Check sheet for the modelled part. Datum: model origin and axes. Units: mm. A direction names the side the tool comes from. Give positions to 0.01 mm unless a question says otherwise; leave off trailing zeros. Loops run counter-clockwise (first coordinate to the right, second up) from the corner with the lowest first, then second, coordinate; pieces in that order, holes last.
```python
from build123d import *

# Parameters (mm, degrees)
SKETCH2_R           = 10
BOSS_EXTRUDE1_DEPTH = 95
BOSS_EXTRUDE2_START = 15
SKETCH3_R           = 10
BOSS_EXTRUDE2_DEPTH = 15
SKETCH5_R           = 2.5
BOSS_EXTRUDE3_DEPTH = 20


with BuildPart() as part:
    # Sketch2 → Boss-Extrude1 (new body)
    with BuildSketch(Plane.XY):
        Circle(SKETCH2_R)
    extrude(amount=BOSS_EXTRUDE1_DEPTH)

    # Sketch3 → Boss-Extrude2 (add)
    with BuildSketch(Plane(origin=(0, 0, 0), x_dir=(-1, 0, 0), z_dir=(0, 0, -1)).offset(BOSS_EXTRUDE2_START)):
        Circle(SKETCH3_R)
    extrude(amount=-BOSS_EXTRUDE2_DEPTH)

    # Sketch5 → Boss-Extrude3 (add)
    with BuildSketch(Plane.XY.offset(95)):
        Circle(SKETCH5_R)
    extrude(amount=BOSS_EXTRUDE3_DEPTH)


solid = part.part
```
(1) Section check D-D on z = 107.5. Record the boundary of the cut face in (x, y), plus the area to 3 significant figures.
(2) Material ranges on line 1 (Z direction, x = 4.25, y = -6); line 2 (Y direction, x = -0.5, z = 34); line 3 (Y direction, x = 1, z = 83), recorded low to high.
(3) Access from +Z, -Z, +X, -X, +Y, -Y to the whole of each face (thin tool, end or side, straight path). Record for faces 1 (the face through (0, 0, -15)), 2 (the face through (-0.54, -2.44, 104.86)).
(4) Section check C-C on z = 86. Record the boundary of the cut face in (x, y).
(5) Section check A-A on x = 0. Record the boundary of the cut face in (y, z), plus the area to 3 significant figures.
(6) Gauge pin test, flat ends, axial feed: pin 1 Ø3 at (y, z) = (-4, 15.5) entering from +X; pin 2 Ø8 at (x, y) = (-6.5, -4) entering from +Z; pin 3 Ø8 at (x, z) = (-6.5, 15.5) entering from -Y. Record the tip position at first contact, or that the pin passes through.
Computed values:
1. outline: circle Ø5 at (0, 0)
1. area: 19.6 mm2
2. line 1: z = -15 to 95
2. line 2: y = -9.99 to 9.99
2. line 3: y = -9.95 to 9.95
3. face 1: -Z, +X, -X, +Y, -Y
3. face 2: +Z
4. outline: circle Ø20 at (0, 0)
5. outline: (-10, -15) - (10, -15) - (10, 95) - (2.5, 95) - (2.5, 115) - (-2.5, 115) - (-2.5, 95) - (-10, 95) - close
5. area: 2,300 mm2
6. pin 1: stops at x = 9.68
6. pin 2: stops at z = 95
6. pin 3: stops at y = -9.68
